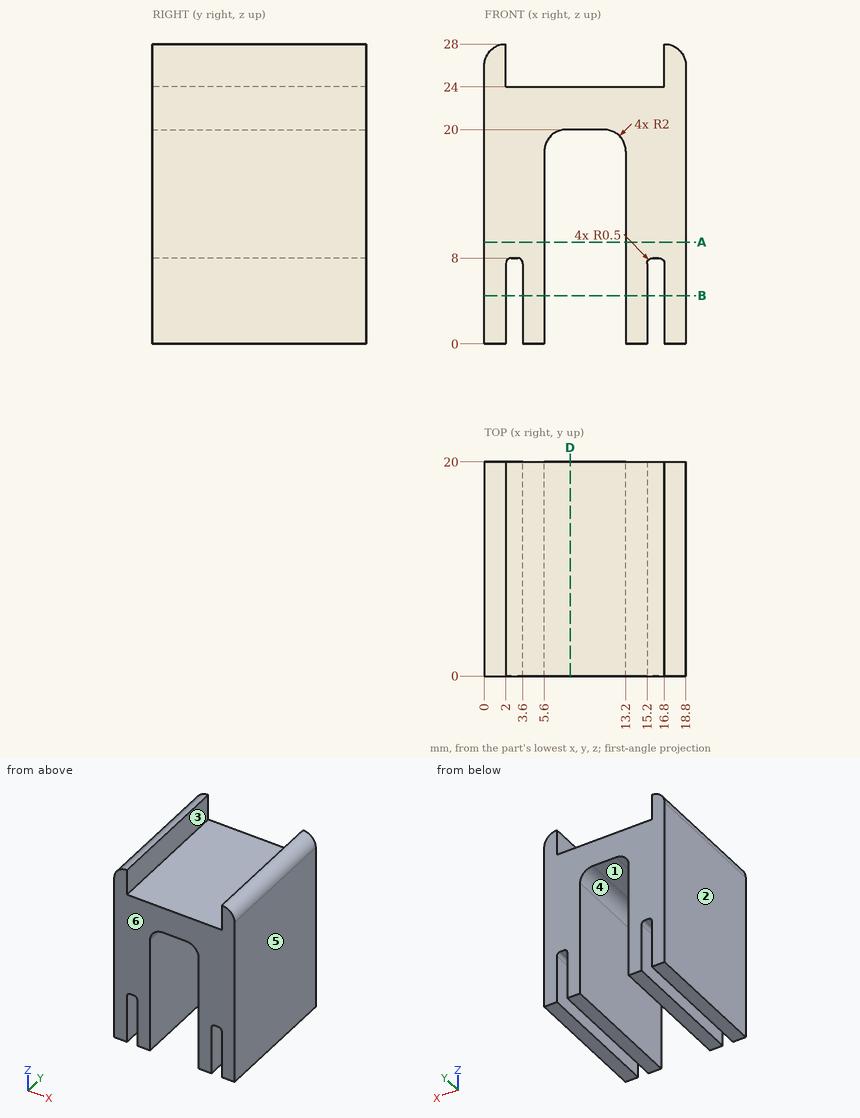
Here's the drawing with two shaded views (mm, measured from the low corner). I have some questions. A direction names the side the tool comes from. Coordinates: 2 decimals unless noted, no trailing zeros. Order: outer loops, then holes, each group sorted by start corner. A loop starts at its lowest first (then second) coordinate and runs counter-clockwise, first axis right, second up. Notation, with made-up numbers: (71, -21) -> (111, -21) arc R15 ccw to (111, -7) -> close; hole circle Ø9 at (-23.75, -21). An arc over 180 degrees is marked (long way). One line per question, with ' | ' between items.
Q1. Thinking about a two-plate mould opening in X: for the marked faces 4, 5 and 6, which applies, pulls with the +X half, pulls with the -X half, needs draft (parallel to the pull), parting line crosses it, or undercut?
Return value:
face 4: undercut | face 5: pulls with the +X half | face 6: needs draft
Q2. Imagine slicing it at D-D on x = 8. Please give me the cut outline in (y, z).
Return value:
outline: (0, 20) -> (20, 20) -> (20, 24) -> (0, 24) -> close
Q3. If I drill on L1, parallel to X at y = 7, z = 3; L2, parallel to X at y = 9.75, z = 24.5; L3, parallel to X at y = 18, z = 16.5, over which ranges is the centre line in solid material (lowest first)?
Return value:
L1: 0 to 2, 3.6 to 5.6, 13.2 to 15.2, 16.8 to 18.8 | L2: 0 to 2, 16.8 to 18.8 | L3: 0 to 5.6, 13.2 to 18.8
Q4. Imagine slicing it at B-B on z = 4.5. Please give me the cut outline in (x, y).
Return value:
outline: (0, 0) -> (2, 0) -> (2, 20) -> (0, 20) -> close; (3.6, 0) -> (5.6, 0) -> (5.6, 20) -> (3.6, 20) -> close; (13.2, 0) -> (15.2, 0) -> (15.2, 20) -> (13.2, 20) -> close; (16.8, 0) -> (18.8, 0) -> (18.8, 20) -> (16.8, 20) -> close
Q5. On a 3-axis mill with a long thin cutter (end or side, diameter ignored), from which of +Z, -Z, +X, -X, +Y, -Y can I reach the whole of each face in a straight line? I mean the marked faces 1, 2 and 3. Say none if no direction works.
Return value:
face 1: -Z, +Y, -Y | face 2: +Z, -Z, -X, +Y, -Y | face 3: +Z, +Y, -Y
Q6. I'm going to push flat-ended pins straight in: P1, Ø7.5, axis at x = 12, y = 6.5, coming from the +Z side; P2, Ø3, axis at x = 9, y = 13, coming from the -Z side; P3, Ø0.7, axis at x = 3, y = 10.5, coming from the -Z side. Where does each tip first touch, or does it pass through?
Return value:
P1: z = 24 | P2: z = 20 | P3: z = 7.93
Q7. Imagine slicing it at A-A on z = 9.5. Please give me the cut outline in (x, y).
Return value:
outline: (0, 0) -> (5.6, 0) -> (5.6, 20) -> (0, 20) -> close; (13.2, 0) -> (18.8, 0) -> (18.8, 20) -> (13.2, 20) -> close
